Autodesk Inventor part; units mm, degrees
ref_plane "YZ Plane" through (0, 0, 0) normal (1, 0, 0) x (0, 1, 0)
ref_plane "XZ Plane" through (0, 0, 0) normal (0, 1, 0) x (-1, 0, 0)
ref_plane "XY Plane" through (0, 0, 0) normal (0, 0, 1) x (1, 0, 0)
sketch "Sketch1" plane through (0, 0, 0) normal (0, 0, 1) x (1, 0, 0)
  arc A0 (-2.4847, -161.9059) -> (161.2805, 14.4329) centre (0, 0) ccw
  line L0 (-2.4847, -161.9059) -> (-2.4847, -174.6059)
  line L1 (175.9176, 141.4329) -> (149.9153, 141.4329)
  line L2 (149.9153, 141.4329) -> (200.7153, 141.4329)
  line L3 (200.7153, 141.4329) -> (200.7153, -174.6059)
  line L4 (149.9153, 141.4329) -> (161.2805, 14.4329)
  line L5 (-2.4847, -161.9224) -> (-2.4847, -174.6059)
  line L6 (200.7153, 141.4329) -> (200.7153, -391.7131)
  line L7 (-2.4847, -174.6059) -> (-2.4847, -417.3671)
  line L8 (-2.4847, -417.3671) -> (175.0613, -417.3671)
  line L9 (200.7153, -417.3671) -> (199.9221, -417.3671)
  line L10 (175.0613, -417.3671) -> (175.0613, -391.7131)
  line L11 (175.0613, -391.7131) -> (200.7153, -391.7131)
  dimension "d1" = 323.85
  dimension "d4" = 50.8
  dimension "d6" = 127
  dimension "d9" = 11.3652
  dimension "d10" = 127.5075
  dimension "d11" = 558.8
  dimension "d14" = 203.2
  dimension "d15" = 25.654
  dimension "d16" = 25.654
extrude "Extrusion1" add sketch "Sketch1" along normal blind 3.175
sketch "Sketch2" plane through (0, 0, 3.175) normal (0, 0, 1) x (1, 0, 0)
  line L0 (200.7153, 141.4329) -> (200.7153, -391.7131)
  line L1 (200.7153, 141.4329) -> (149.9153, 141.4329)
  point P0 (0, 0)
  point P1 (188.0153, 116.0329)
  point P2 (188.0153, 39.8329)
  point P3 (188.0153, -36.3671)
  point P4 (188.0153, -112.5671)
  point P5 (188.0153, -188.7671)
  point P6 (188.0153, -264.9671)
  point P7 (188.0153, -341.1671)
  dimension "d19" = 12.7
  dimension "d20" = 12.7
  dimension "d21" = 12.7
  dimension "d22" = 12.7
  dimension "d23" = 12.7
  dimension "d24" = 12.7
  dimension "d25" = 76.2
  dimension "d26" = 76.2
  dimension "d27" = 76.2
  dimension "d28" = 76.2
  dimension "d29" = 76.2
  dimension "d30" = 76.2
  dimension "d31" = 25.4
hole "Hole1" at (188.0153, 116.0329, 3.175) at (188.0153, 39.8329, 3.175) at (188.0153, -36.3671, 3.175) at (188.0153, -112.5671, 3.175) at (188.0153, -188.7671, 3.175) at (188.0153, -264.9671, 3.175) at (188.0153, -341.1671, 3.175) direction (0, 0, -1) diameter 7.1374 end through all
sketch "Sketch3" plane through (0, 0, 3.175) normal (0, 0, 1) x (1, 0, 0)
  line L0 (-2.4847, -161.9059) -> (-2.4847, -417.3671)
  line L1 (-2.4847, -417.3671) -> (175.0613, -417.3671)
  point P0 (0, 0)
  point P1 (22.9153, -188.7671)
  point P2 (22.9153, -264.9671)
  point P3 (22.9153, -341.1671)
  dimension "d39" = 25.4
  dimension "d40" = 25.4
  dimension "d41" = 25.4
  dimension "d42" = 76.2
  dimension "d43" = 76.2
  dimension "d44" = 76.2
hole "Hole2" at (22.9153, -188.7671, 3.175) at (22.9153, -264.9671, 3.175) at (22.9153, -341.1671, 3.175) direction (0, 0, -1) diameter 7.1374 end through all
sketch "Sketch4" plane through (0, 0, 3.175) normal (0, 0, 1) x (1, 0, 0)
  line L0 (-2.4847, -417.3671) -> (175.0613, -417.3671)
  line L1 (-2.4847, -161.9059) -> (-2.4847, -417.3671)
  line L2 (162.6153, -417.3671) -> (-2.4847, -417.3671)
  line L3 (-2.4847, -417.3671) -> (-2.4847, -285.2871)
  line L4 (-2.4847, -285.2871) -> (162.6153, -285.2871)
  line L5 (162.6153, -285.2871) -> (162.6153, -417.3671)
  line L6 (175.0613, -417.3671) -> (175.0613, -391.7131)
  line L7 (175.0613, -391.7131) -> (200.7153, -391.7131)
  line L8 (200.7153, -391.7131) -> (200.7153, 141.4329)
  circle A0 centre (22.9153, -341.1671) radius 3.5687
  circle A1 centre (22.9153, -264.9671) radius 3.5687
  point P0 (0, 0)
  dimension "d52" = 132.08
  dimension "d53" = 38.1
extrude "Extrusion2" cut sketch "Sketch4" against normal blind 25.4 contours L1 L4 L5 L0
properties part number "LauncherSidePlate"
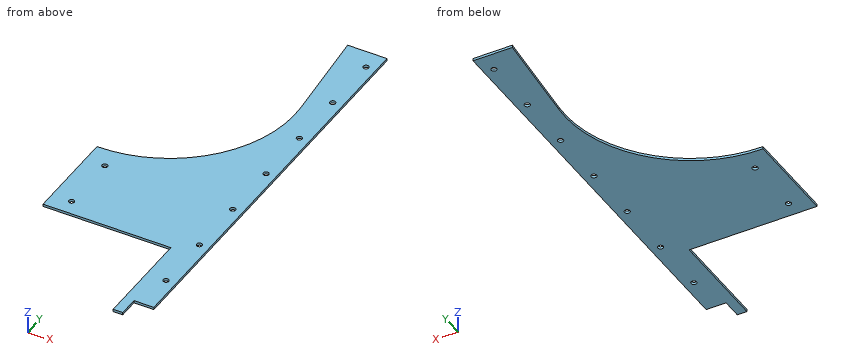
Design review of the part built by this model. Coordinates are the model's own, in mm. Round coordinates to 2 decimals unless told otherwise and drop trailing zeros. Order: outer loops, then holes, each group sorted by start corner. A loop starts at its lowest first (then second) coordinate and runs counter-clockwise, first axis right, second up.
1) Consider section A-A (z = 1.65). Count the separate pieces of the cut face and the enclosed holes in it, plus the area to 3 significant figures.
The answers:
separate pieces: 1
enclosed holes: 9
area: 47,300 mm2
2) Consider section C-C (y = 66). State the section outline as (x, z) points (3 decimals), plus the area to 3 significant figures.
The answers:
outline: (156.666, 0) - (200.715, 0) - (200.715, 3.175) - (156.666, 3.175) - close
area: 140 mm2
3) For L1, parallel to X at y = -0.5, z = 2.25; L2, parallel to X at y = -326, z = 0.65; L3, parallel to Y at x = 87.5, z = 2.15, list the stretches that pass through material, from the lowest coordinate up.
The answers:
L1: x = 161.92 to 200.72
L2: x = 162.62 to 200.72
L3: y = -285.29 to -136.25
4) Clearance check with flat-ended pins moving along their axes: pin 1 Ø1 at (x, z) = (191, 1) entering from -Y; pin 2 Ø1 at (x, z) = (95.5, 2) entering from -Y; pin 3 Ø1.6 at (y, z) = (-403.5, 1.5) entering from +X; pin 4 Ø5.5 at (x, y) = (22.92, -264.97) entering from -Z. State where each tip first meets the part, or that it passes through.
The answers:
pin 1: stops at y = -391.71
pin 2: stops at y = -285.29
pin 3: stops at x = 175.06
pin 4: passes through
5) Consider section B-B (x = 53). State the section outline as (y, z) points (3 decimals), plus the area to 3 significant figures.
The answers:
outline: (-285.287, 0) - (-153.006, 0) - (-153.006, 3.175) - (-285.287, 3.175) - close
area: 420 mm2
